```python
from build123d import *

# Parameters (mm, degrees)
SKETCH_2_R      = 5.5
SKETCH_2_R_2    = 5
SKETCH_2_R_3    = 1.65
EXTRUDE_1_DEPTH = 5


with BuildPart() as part:
    # 草图2 → 凸台-拉伸1 (new body)
    with BuildSketch(Plane.XY):
        with BuildLine():
            Line((1.3125, 17.450711841), (100.75, 9.971835338))
            ThreePointArc((100.75, 9.971835338), (110, 0), (100.75, -9.971835338))
            Line((100.75, -9.971835338), (1.3125, -17.450711841))
            ThreePointArc((1.3125, -17.450711841), (-17.5, 0), (1.3125, 17.450711841))
        make_face()
        Circle(SKETCH_2_R, mode=Mode.SUBTRACT)
        with Locations((100, 0)):
            Circle(SKETCH_2_R_2, mode=Mode.SUBTRACT)
        with Locations((0, 13)):
            Circle(SKETCH_2_R_3, mode=Mode.SUBTRACT)
        with Locations((13, 0)):
            Circle(SKETCH_2_R_3, mode=Mode.SUBTRACT)
        with Locations((0, -13)):
            Circle(SKETCH_2_R_3, mode=Mode.SUBTRACT)
        with Locations((-13, 0)):
            Circle(SKETCH_2_R_3, mode=Mode.SUBTRACT)
        with BuildLine():
            Line((17.322897462, -11.232418418), (48.094795732, -8.918007587))
            ThreePointArc((48.094795732, -8.918007587), (49.411083562, -8.283787571), (49.944795732, -6.92364052))
            Line((49.944795732, -6.92364052), (49.944795732, 6.92364052))
            ThreePointArc((49.944795732, 6.92364052), (49.411083562, 8.283787571), (48.094795732, 8.918007587))
            Line((48.094795732, 8.918007587), (17.322897462, 11.232418418))
            ThreePointArc((17.322897462, 11.232418418), (15.495779502, 10.327673003), (15.411574646, 8.290558904))
            ThreePointArc((15.411574646, 8.290558904), (17.5, 0), (15.411574646, -8.290558904))
            ThreePointArc((15.411574646, -8.290558904), (15.495779502, -10.327673003), (17.322897462, -11.232418418))
        make_face(mode=Mode.SUBTRACT)
        with BuildLine():
            Line((57.094795732, 8.241101103), (88.788774342, 5.857338922))
            ThreePointArc((88.788774342, 5.857338922), (90.307315813, 4.965681861), (90.532311952, 3.219143212))
            ThreePointArc((90.532311952, 3.219143212), (90, 0), (90.532311952, -3.219143212))
            ThreePointArc((90.532311952, -3.219143212), (90.307315813, -4.965681861), (88.788774342, -5.857338922))
            Line((88.788774342, -5.857338922), (57.094795732, -8.241101103))
            ThreePointArc((57.094795732, -8.241101103), (55.584648681, -7.713021866), (54.944795732, -6.246734036))
            Line((54.944795732, -6.246734036), (54.944795732, 6.246734036))
            ThreePointArc((54.944795732, 6.246734036), (55.584648681, 7.713021866), (57.094795732, 8.241101103))
        make_face(mode=Mode.SUBTRACT)
    extrude(amount=EXTRUDE_1_DEPTH)


solid = part.part
```
Can you work these out from the model? Positions are in its coordinate system, mm. A direction names the side the tool comes from. Round coordinates to 2 decimals unless told otherwise and drop trailing zeros. Loops run counter-clockwise (first coordinate to the right, second up) from the corner with the lowest first, then second, coordinate; pieces in that order, holes last.
Item 1: Suppose I cut it at A-A, the plane z = 3.75. State how many separate pieces and enclosed holes the cut face has, then the cut area to 3 significant figures.
Item 2: Please list where these lines run through material, in increasing order: L1, parallel to Y at x = 1, z = 4.85; L2, parallel to Y at x = 41.5, z = 1.2; L3, parallel to Y at x = 70, z = 4.3.
Item 3: Suppose I cut it at D-D, the plane y = -13. Write out the boundary of the cut face in (x, z), then the cut area to 3 significant figures.
Item 4: Suppose I cut it at C-C, the plane x = 84. Write out the boundary of the cut face in (y, z).
Item 5: Which directions (+Z, -Z, +X, -X, +Y, -Y) give clear straight access to the entire face, cutting with the end or side of a thin tool? Please do faces 4 (the flat face through (50.335, 13.764, 2.465)), 5 (the flat face through (49.945, 0, 2)).
Item 6: Will these pins go through, and if not, where does the flat tip stop? pin 1 Ø2 at (y, z) = (10.5, 2) entering from -X; pin 2 Ø2 at (x, y) = (0, -13) entering from -Z; pin 3 Ø2 at (x, z) = (93, 4.5) entering from +Y; pin 4 Ø3 at (y, z) = (6, 4) entering from -X.
Item 7: If we mould it in two halves opening along X, with no side actions, what happens to faces 1 (the flat face through (33, -11, 0)), 2 (the flat face through (51.73, -13.66, 2.46)), 3 (the cylindrical face through (-1.19, -5.37, 2.46))? For each: +X half, -X half, draft (parallel to the pull), parting line (faces both ways), or undercut.
Item 8: Suppose I cut it at B-B, the plane y = 0. Write out the boundary of the cut face in (x, z).
Reported:
1. separate pieces: 1
1. enclosed holes: 8
1. area: 2,020 mm2
2. L1: y = -17.47 to -14.31, -11.69 to -5.41, 5.41 to 11.69, 14.31 to 17.47
2. L2: y = -14.43 to -9.41, 9.41 to 14.43
2. L3: y = -12.28 to -7.27, 7.27 to 12.28
3. outline: (-11.72, 0) - (-1.65, 0) - (-1.65, 5) - (-11.72, 5) - close; (1.65, 0) - (60.49, 0) - (60.49, 5) - (1.65, 5) - close
3. area: 345 mm2
4. outline: (-11.23, 0) - (-6.22, 0) - (-6.22, 5) - (-11.23, 5) - close; (6.22, 0) - (11.23, 0) - (11.23, 5) - (6.22, 5) - close
5. face 4: +Z, -Z, +X, +Y
5. face 5: +Z, -Z
6. pin 1: stops at x = -14.7
6. pin 2: passes through
6. pin 3: stops at y = 10.63
6. pin 4: stops at x = -16.91
7. face 1: draft
7. face 2: +X half
7. face 3: undercut
8. outline: (-17.5, 0) - (-14.65, 0) - (-14.65, 5) - (-17.5, 5) - close; (-11.35, 0) - (-5.5, 0) - (-5.5, 5) - (-11.35, 5) - close; (5.5, 0) - (11.35, 0) - (11.35, 5) - (5.5, 5) - close; (14.65, 0) - (17.5, 0) - (17.5, 5) - (14.65, 5) - close; (49.94, 0) - (54.94, 0) - (54.94, 5) - (49.94, 5) - close; (90, 0) - (95, 0) - (95, 5) - (90, 5) - close; (105, 0) - (110, 0) - (110, 5) - (105, 5) - close
